Here's how the part is built. I have some questions about the finished solid (model axes, mm). A direction names the side the tool comes from. Round coordinates to 2 decimals unless told otherwise and drop trailing zeros. Order: outer loops, then holes, each group sorted by start corner. A loop starts at its lowest first (then second) coordinate and runs counter-clockwise, first axis right, second up. Notation, with made-up numbers: (54, -29) -> (98, -29) arc R14 cw to (98, -4) -> close; hole circle Ø11 at (41, 58). An arc over 180 degrees is marked (long way). Use a Markdown table: item, result. Add a question column.
(1) On a 3-axis mill with a long thin cutter (end or side, diameter ignored), from which of +Z, -Z, +X, -X, +Y, -Y can I reach the whole of each face in a straight line? I mean faces 1 (the face through (-17.6, 5.8, 8.8)), 2 (the face through (14, 4.1, 7)), 3 (the face through (-10, 1, 0)). Say none if no direction works.
(2) I want a section at B-B, the plane y = 0.5. Please give me the cut outline in (x, z), then the cut area to 3 significant figures.
(3) I'm going to push flat-ended pins straight in: P1, Ø6, axis at x = 2, z = -4, coming from the +Y side; P2, Ø8, axis at x = 6.5, z = -5, coming from the -Y side; P3, Ø4.5, axis at x = 14, z = 8, coming from the +Y side. Where does each tip first touch, or does it pass through?
(4) I want a section at A-A, the plane z = 3. Please give me the cut outline in (x, y), then the cut area to 3 significant figures.
(5) I want a section at C-C, the plane x = 14.2. Please give me the cut outline in (y, z), then the cut area to 3 significant figures.
(6) I want a section at D-D, the plane y = 6. Please give me the cut outline in (x, z).
(7) Thinking about a two-plate mould opening in Z: for faces 4 (the face through (-19, 7.6, -9)), 5 (the face through (10, 1, 0)), 6 (the face through (-19.715, 2.079, 10.049)), which applies, pulls with the +Z half, pulls with the -Z half, needs draft (parallel to the pull), parting line crosses it, or undercut?
(8) If I drill on probe 1 along X at (y, z) = (3, -8.75); probe 2 along Z at (x, y) = (-3, 1); probe 3 along X at (y, z) = (1.4, 8.75), over which ranges is the centre line in solid material (lowest first)?
from build123d import *

# Parameters (mm, degrees)
SKETCH1_W           = 40
SKETCH1_H           = 20.7
BOSS_EXTRUDE1_DEPTH = 4.1
SKETCH2_R           = 1.2
BOSS_EXTRUDE2_DEPTH = 3.5
SKETCH3_R           = 1.3
CUT_EXTRUDE1_DEPTH  = 23.889571861
FILLET1_R           = 1
SKETCH4_W           = 48.8996316
SKETCH4_H           = 28.322761229
SKETCH4_R           = 2.5
CUT_EXTRUDE2_DEPTH  = 1.5
SKETCH5_W           = 20
SKETCH5_H           = 8
CUT_EXTRUDE3_DEPTH  = 24.067780561


with BuildPart() as part:
    # Sketch1 → Boss-Extrude1 (new body)
    with BuildSketch(Plane(origin=(0, 0, 0), x_dir=(1, 0, 0), z_dir=(0, 1, 0))):
        Rectangle(SKETCH1_W, SKETCH1_H)
    extrude(amount=BOSS_EXTRUDE1_DEPTH)

    # Sketch2 → Boss-Extrude2 (add)
    with BuildSketch(Plane(origin=(0, 4.1, 0), x_dir=(1, 0, 0), z_dir=(0, 1, 0))):
        with Locations(Location((-18.8, 8.75, 0), (0, 0, 180))):
            Circle(SKETCH2_R)
        with Locations(Location((-18.8, -8.75, 0), (0, 0, 180))):
            Circle(SKETCH2_R)
    extrude(amount=BOSS_EXTRUDE2_DEPTH)

    # Sketch3 → Cut-Extrude1 (cut, through all)
    with BuildSketch(Plane(origin=(0, 4.1, 0), x_dir=(1, 0, 0), z_dir=(0, 1, 0))):
        with Locations(Location((14.2, 8.75, 0), (0, 0, 270))):
            Circle(SKETCH3_R)
        with Locations(Location((14.2, -8.75, 0), (0, 0, 270))):
            Circle(SKETCH3_R)
    extrude(amount=-CUT_EXTRUDE1_DEPTH, mode=Mode.SUBTRACT)

    # Fillet1
    fillet1_edges = [part.edges().sort_by_distance(p)[0] for p in [
        (20, 2.05, 10.35),
        (-20, 2.05, 10.35),
        (-20, 2.05, -10.35),
        (20, 2.05, -10.35),
    ]]
    fillet(fillet1_edges, radius=FILLET1_R)

    # Sketch4 → Cut-Extrude2 (cut)
    with BuildSketch(Plane(origin=(0, 4.1, 0), x_dir=(1, 0, 0), z_dir=(0, 1, 0))):
        with Locations((0.354773627, -0.266080221)):
            Rectangle(SKETCH4_W, SKETCH4_H)
        with Locations((-18.8, 8.75)):
            Circle(SKETCH4_R, mode=Mode.SUBTRACT)
        with Locations((-18.8, -8.75)):
            Circle(SKETCH4_R, mode=Mode.SUBTRACT)
        with Locations((14.2, -8.75)):
            Circle(SKETCH4_R, mode=Mode.SUBTRACT)
        with Locations((14.2, 8.75)):
            Circle(SKETCH4_R, mode=Mode.SUBTRACT)
    extrude(amount=-CUT_EXTRUDE2_DEPTH, mode=Mode.SUBTRACT)

    # Sketch5 → Cut-Extrude3 (cut, through all)
    with BuildSketch(Plane(origin=(0, 2.6, 0), x_dir=(1, 0, 0), z_dir=(0, 1, 0))):
        Rectangle(SKETCH5_W, SKETCH5_H)
    extrude(amount=-CUT_EXTRUDE3_DEPTH, mode=Mode.SUBTRACT)


solid = part.part
Taken from the geometry:
| question | item | result |
|---|---|---|
| 1 | face 1 | +Y |
| 1 | face 2 | +Z, -Z, +X, +Y |
| 1 | face 3 | +Y, -Y |
| 2 | outline | (-20, -9.35) arc R1 ccw to (-19, -10.35) -> (19, -10.35) arc R1 ccw to (20, -9.35) -> (20, 9.35) arc R1 ccw to (19, 10.35) -> (-19, 10.35) arc R1 ccw to (-20, 9.35) -> close; hole (-10, -4) -> (10, -4) -> (10, 4) -> (-10, 4) -> close; hole circle Ø2.6 at (14.2, -8.75); hole circle Ø2.6 at (14.2, 8.75) |
| 2 | area | 657 mm2 |
| 3 | P1 | stops at y = 2.6 |
| 3 | P2 | stops at y = 0 |
| 3 | P3 | stops at y = 4.1 |
| 4 | outline | (-20, 0) -> (-10, 0) -> (-10, 2.6) -> (-20, 2.6) -> close; (10, 0) -> (20, 0) -> (20, 2.6) -> (10, 2.6) -> close |
| 4 | area | 52.0 mm2 |
| 5 | outline | (0, -10.35) -> (4.1, -10.35) -> (4.1, -10.05) -> (0, -10.05) -> close; (0, -7.45) -> (4.1, -7.45) -> (4.1, -6.25) -> (2.6, -6.25) -> (2.6, 6.25) -> (4.1, 6.25) -> (4.1, 7.45) -> (0, 7.45) -> close; (0, 10.05) -> (4.1, 10.05) -> (4.1, 10.35) -> (0, 10.35) -> close |
| 5 | area | 44.8 mm2 |
| 6 | outline | circle Ø2.4 at (-18.8, -8.75); circle Ø2.4 at (-18.8, 8.75) |
| 7 | face 4 | needs draft |
| 7 | face 5 | undercut |
| 7 | face 6 | pulls with the +Z half |
| 8 | probe 1 | x = -20 to -16.3, 11.7 to 12.9, 15.5 to 16.7 |
| 8 | probe 2 | z = -10.35 to -4, 4 to 10.35 |
| 8 | probe 3 | x = -20 to 12.9, 15.5 to 20 |
